Autodesk Inventor part; units mm, degrees
ref_plane "YZ Plane" through (0, 0, 0) normal (1, 0, 0) x (0, 1, 0)
ref_plane "XZ Plane" through (0, 0, 0) normal (0, 1, 0) x (-1, 0, 0)
ref_plane "XY Plane" through (0, 0, 0) normal (0, 0, 1) x (1, 0, 0)
sketch "Sketch1" plane through (0, 0, 0) normal (0, 0, 1) x (1, 0, 0)
  line L0 (0, 0) -> (25.4, 0)
  line L1 (25.4, 0) -> (25.4, -50.8)
  line L2 (25.4, -50.8) -> (0, -50.8)
  line L3 (0, -50.8) -> (0, 0)
  line L4 (22.225, -3.175) -> (3.175, -3.175)
  line L5 (3.175, -3.175) -> (3.175, -47.625)
  line L6 (3.175, -47.625) -> (22.225, -47.625)
  line L7 (22.225, -47.625) -> (22.225, -3.175)
  dimension "d0" = 25.4
  dimension "d1" = 50.8
  dimension "d2" = 3.175
extrude "Extrusion1" add sketch "Sketch1" along normal blind 381
sketch "Sketch2" plane through (25.4, -50.8, 0) normal (1, 0, 0) x (0, 0, -1)
  circle A0 centre (-355.6, 25.4) radius 14.2875
  circle A1 centre (-203.2, 25.4) radius 14.2875
  circle A2 centre (-50.8, 25.4) radius 14.2875
  line L0 (0, 0) -> (-381, 0)
  line L1 (0, 50.8) -> (-381, 50.8)
  line L2 (0, 50.8) -> (0, 0)
  dimension "d6" = 28.575
  dimension "d7" = 28.575
  dimension "d8" = 28.575
  dimension "d10" = 25.4
  dimension "d11" = 25.4
  dimension "d12" = 25.4
  dimension "d13" = 50.8
  dimension "d14" = 152.4
  dimension "d15" = 152.4
extrude "Extrusion2" cut sketch "Sketch2" against normal blind 381
sketch "Sketch3" plane through (0, -50.8, 0) normal (-1, 0, 0) x (0, 0, 1)
  circle A0 centre (127, 25.4) radius 14.2875
  circle A1 centre (279.4, 25.4) radius 14.2875
  line L0 (0, 0) -> (381, 0)
  circle A2 centre (203.2, 25.4) radius 14.2875
  circle A3 centre (355.6, 25.4) radius 14.2875
  point P0 (0, 50.8)
  dimension "d19" = 28.575
  dimension "d20" = 28.575
  dimension "d21" = 25.4
  dimension "d22" = 25.4
  dimension "d23" = 76.2
  dimension "d24" = 76.2
  dimension "d25" = 76.2
extrude "Extrusion3" cut sketch "Sketch3" against normal blind 25.4 contours A0 | A1
properties part number "intake 1"
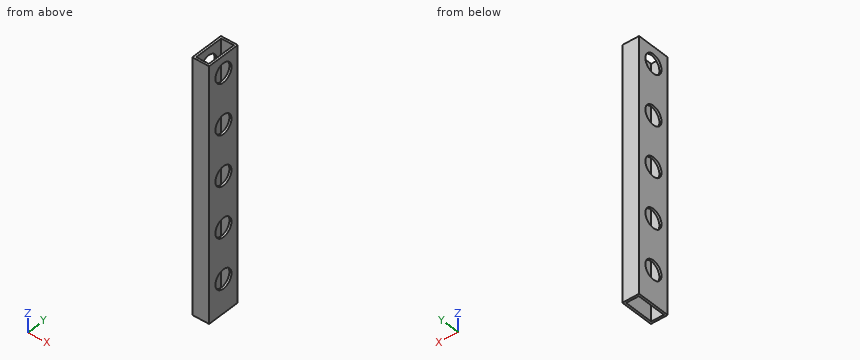
Here's how the part is built. I have some questions about the finished solid (model axes, mm). Round coordinates to 2 decimals unless told otherwise and drop trailing zeros. Loops run counter-clockwise (first coordinate to the right, second up) from the corner with the lowest first, then second, coordinate; pieces in that order, holes last. Notation, with made-up numbers: (75.25, -5.5) -> (99.25, -5.5) arc R18 ccw to (99.25, 10.5) -> close; hole circle Ø11 at (38.25, 31.5). An arc over 180 degrees is marked (long way). Answer as CSV lines item,"result". Start each with the question number.
1. Imagine slicing it at B-B on z = 150. Write out the boundary of the cut face in (x, y) (3 decimals), plus the area to 3 significant figures.
2. Imagine slicing it at D-D on y = -25.4. State how many separate pieces and enclosed holes the cut face has, plus the area to 3 significant figures.
3. Imagine slicing it at C-C on z = 355.6. Write out the boundary of the cut face in (x, y) (1 decimal), plus the area to 3 significant figures.
4. Imagine slicing it at A-A on x = 7. Write out the boundary of the cut face in (y, z) (3 decimals), plus the area to 3 significant figures.
5. I'm going to push a flat-ended pin straight in: P1, Ø9.5, axis at x = 12.5, z = 272.5, coming from the +Y side. Where does the tip first touch, or does it pass through?
6. I need wall thicknesses on probe 1 along X at (y, z) = (-28.5, 311) (3 decimals); probe 2 along Y at (x, z) = (7.75, 65.5) (3 decimals); probe 3 along Y at (x, z) = (23.7, 279.4). Which ranges of each line are inside material? Lowest first, please. Write a range as from..to.
Solution:
1,outline,"(0, -50.8) -> (25.4, -50.8) -> (25.4, 0) -> (0, 0) -> close; hole (3.175, -47.625) -> (22.225, -47.625) -> (22.225, -3.175) -> (3.175, -3.175) -> close"
1,area,"444 mm²"
2,separate pieces,"12"
2,enclosed holes,"0"
2,area,"1,510 mm²"
3,outline,"(0, -50.8) -> (25.4, -50.8) -> (25.4, -39.7) -> (22.2, -39.7) -> (22.2, -47.6) -> (3.2, -47.6) -> (3.2, -39.7) -> (0, -39.7) -> close; (0, -11.1) -> (3.2, -11.1) -> (3.2, -3.2) -> (22.2, -3.2) -> (22.2, -11.1) -> (25.4, -11.1) -> (25.4, 0) -> (0, 0) -> close"
3,area,"262 mm²"
4,outline,"(-50.8, 0) -> (-47.625, 0) -> (-47.625, 381) -> (-50.8, 381) -> close; (-3.175, 0) -> (0, 0) -> (0, 381) -> (-3.175, 381) -> close"
4,area,"2,420 mm²"
5,P1,"y = 0"
6,probe 1,"0..3.175, 22.225..25.4"
6,probe 2,"-50.8..-47.625, -3.175..0"
6,probe 3,"-50.8..-39.69, -11.11..0"
